Answer from the drawing. Dimensions are ordinates in mm from the lowest x, y and z of the part. A direction names the side the tool comes from. Give positions to 0.01 mm unless a question says otherwise; leave off trailing zeros. Loops run counter-clockwise (first coordinate to the right, second up) from the corner with the lowest first, then second, coordinate; pieces in that order, holes last. Notation, with made-up numbers: (10.5, 12) - (53.5, 12) arc R29 ccw to (53.5, 38) - close; hole circle Ø10 at (31.5, 80). An arc over 180 degrees is marked (long way). Put each result on its own line as item: value. Start each with the question number.
1. A cutting plane is placed at B-B, the plane y = 2.5. Determine the outline of the cut face in (x, z), plus the area to 3 significant figures.
2. Consider L1, parallel to X at y = 2.5, z = 0.75; L2, parallel to Y at x = 13.45, z = 0.6; L3, parallel to Y at x = 0.5, z = 0.95. Determine where each line is inside the solid, lowest interval first. Write a range as from..to.
3. For the marked faces 1, 2 and 3, determine the directions among +Z, -Z, +X, -X, +Y, -Y from which every point of the face is accessible in a straight line to the end or side of a thin tool.
4. For a pull along Y with two mould halves and no side action, classify the marked faces 4, 5 and 6 as released by +Y, released by -Y, zero draft, split by the parting line, or undercut.
5. Given pin 1 Ø1.1 at (x, y) = (13.45, 2.5) entering from -Z; pin 2 Ø0.6 at (x, z) = (15, 1) entering from -Y; pin 3 Ø1 at (x, z) = (1, 1) entering from +Y, each flat-ended and moving along its own axis, determine where each tip first touches the part or whether it passes through.
6. A cutting plane is placed at C-C, the plane z = 0.55. Determine the outline of the cut face in (x, y).
7. A cutting plane is placed at A-A, the plane x = 2.75. Determine the outline of the cut face in (y, z).
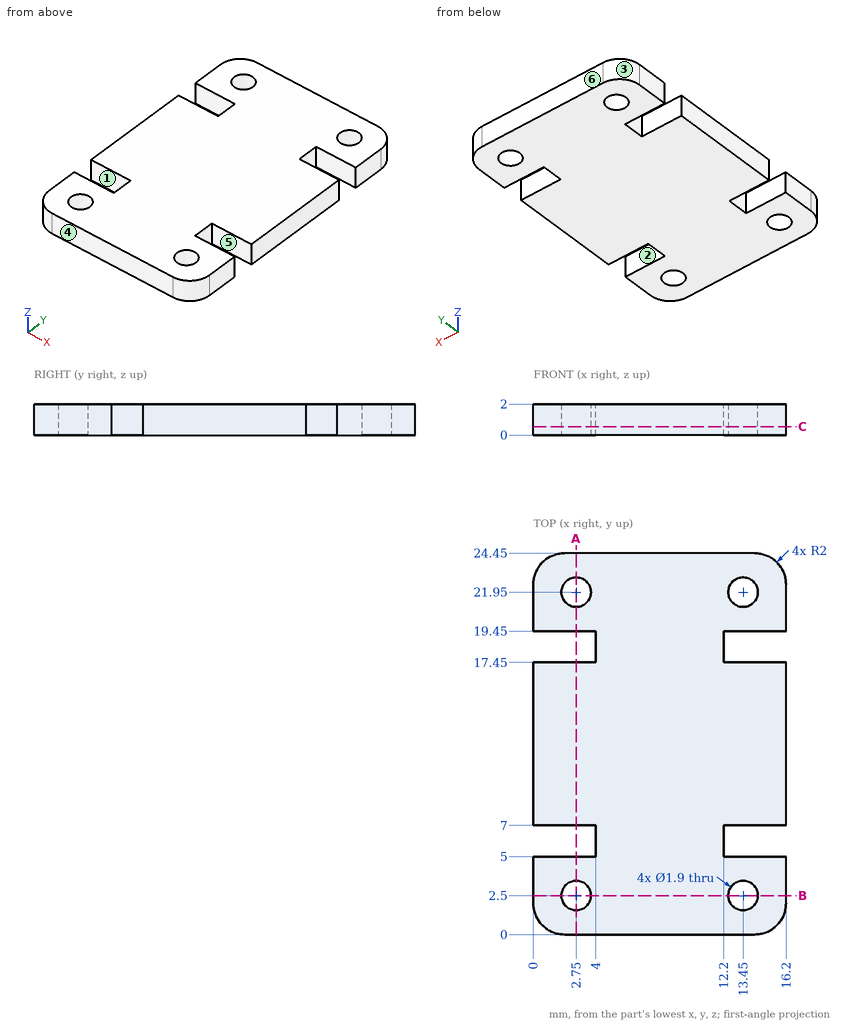
Return value:
1. outline: (0, 0) - (1.8, 0) - (1.8, 2) - (0, 2) - close; (3.7, 0) - (12.5, 0) - (12.5, 2) - (3.7, 2) - close; (14.4, 0) - (16.2, 0) - (16.2, 2) - (14.4, 2) - close
1. area: 24.8 mm2
2. L1: x = 0..1.8, 3.7..12.5, 14.4..16.2
2. L2: y = 0..1.55, 3.45..5, 7..17.45, 19.45..21, 22.9..24.45
2. L3: y = 0.68..5, 7..17.45, 19.45..23.77
3. face 1: +Z, -Z, -X
3. face 2: +Z, -Z, +X
3. face 3: +Z, -Z, -X, +Y
4. face 4: released by -Y
4. face 5: undercut
4. face 6: released by +Y
5. pin 1: passes through
5. pin 2: stops at y = 0.06
5. pin 3: stops at y = 24.39
6. outline: (0, 2) arc R2 ccw to (2, 0) - (14.2, 0) arc R2 ccw to (16.2, 2) - (16.2, 5) - (12.2, 5) - (12.2, 7) - (16.2, 7) - (16.2, 17.45) - (12.2, 17.45) - (12.2, 19.45) - (16.2, 19.45) - (16.2, 22.45) arc R2 ccw to (14.2, 24.45) - (2, 24.45) arc R2 ccw to (0, 22.45) - (0, 19.45) - (4, 19.45) - (4, 17.45) - (0, 17.45) - (0, 7) - (4, 7) - (4, 5) - (0, 5) - close; hole circle Ø1.9 at (2.75, 2.5); hole circle Ø1.9 at (2.75, 21.95); hole circle Ø1.9 at (13.45, 2.5); hole circle Ø1.9 at (13.45, 21.95)
7. outline: (0, 0) - (1.55, 0) - (1.55, 2) - (0, 2) - close; (3.45, 0) - (5, 0) - (5, 2) - (3.45, 2) - close; (7, 0) - (17.45, 0) - (17.45, 2) - (7, 2) - close; (19.45, 0) - (21, 0) - (21, 2) - (19.45, 2) - close; (22.9, 0) - (24.45, 0) - (24.45, 2) - (22.9, 2) - close
